Source: CAD feature listing. Evaluate the final solid. Frame: model axes, mm. Face numbers are marked on the shaded views. A direction names the side the tool comes from. Coordinates: 2 decimals unless noted, no trailing zeros. Order: outer loops, then holes, each group sorted by start corner. A loop starts at its lowest first (then second) coordinate and runs counter-clockwise, first axis right, second up. Notation, with made-up numbers: (49, 28.25) - (85, 28.25) arc R31 cw to (85, 54.25) - close; hole circle Ø8 at (32, 21.5). An arc over 180 degrees is marked (long way). One line per question, with ' | ' between items.
Autodesk Inventor part; units mm, degrees
ref_plane "YZ Plane" through (0, 0, 0) normal (1, 0, 0) x (0, 1, 0)
ref_plane "XZ Plane" through (0, 0, 0) normal (0, 1, 0) x (-1, 0, 0)
ref_plane "XY Plane" through (0, 0, 0) normal (0, 0, 1) x (1, 0, 0)
sketch "Sketch2" plane through (0, 0, 0) normal (0, 0, 1) x (1, 0, 0)
  line L0 (4.2, -19.2857) -> (4.2, 20.7143)
  line L1 (4.2, -19.2857) -> (15, -19.2857)
  line L2 (15, -19.2857) -> (15, -8.3281)
  line L3 (15, -8.3281) -> (20.3713, -0.6476)
  line L4 (20.3713, -0.6476) -> (20.3713, 40.7143)
  line L5 (20.3713, 40.7143) -> (0, 40.7143)
  line L6 (0, 40.7143) -> (0, 20.7143)
  line L7 (0, 20.7143) -> (4.2, 20.7143)
  point P0 (0, 0)
  dimension "d3" = 4.2
  dimension "d4" = 10.8
  dimension "d5" = 60
  dimension "d6" = 20
revolve "Revolution1" add sketch "Sketch2" angle 360 about axis through (0, 40.7143, 0) along (0, -1, 0)
fillet "Fillet1" radius 6 2 edges at (-20.3713, -0.6476, 0) (-15, -8.3281, 0)
fillet "Fillet2" radius 5 1 edges at (-20.3713, 40.7143, 0)
properties part number "Top Knob"
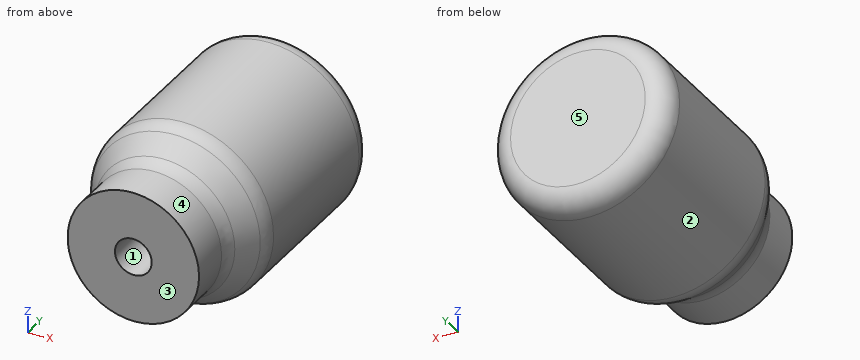
(1) Pull-direction query (Z, two-part tool) for the marked faces 1, 2 and 3; classes: pulls with the +Z half, pulls with the -Z half, needs draft (parallel to the pull), parting line crosses it, or undercut.
Taken from the geometry:
face 1: undercut | face 2: parting line crosses it | face 3: needs draft
(2) Material intervals for L1, parallel to Z at x = 0, y = -10; L2, parallel to Z at x = 0, y = 5; L3, parallel to X at y = -1, z = 2.5, sorted ascending. Write a range as from..to.
Taken from the geometry:
L1: z = -15..-4.2, 4.2..15 | L2: z = -20.37..-4.2, 4.2..20.37 | L3: x = -19.78..-3.37, 3.37..19.78
(3) Cut plane B-B (y = 33.5). Return the cut outline in (x, z).
Taken from the geometry:
outline: circle Ø40.74 at (0, 0)
(4) Set-up query: the marked faces 4 and 5. Return all of +Z, -Z, +X, -X, +Y, -Y with unobstructed straight access to the full face (end or side cutting, diameter ignored); none if empty.
Taken from the geometry:
face 4: -Y | face 5: +Z, -Z, +X, -X, +Y
(5) Pin query (flat end, axial travel): P1, Ø8, axis at x = -15, y = -5, coming from the -Z side; P2, Ø6.5, axis at x = 0, z = 0, coming from the -Y side; P3, Ø8, axis at y = -8, z = -3, coming from the -X side. Return the tip coordinate at first contact, or that it passes through.
Taken from the geometry:
P1: stops at z = -14.99 | P2: stops at y = 20.71 | P3: stops at x = -17.84
(6) Cut plane C-C (y = 8.5). Return the cut outline in (x, z).
Taken from the geometry:
outline: circle Ø40.74 at (0, 0); hole circle Ø8.4 at (0, 0)
(7) Cut plane A-A (y = -12). Return the cut outline in (x, z), and give its area (3 significant figures).
Taken from the geometry:
outline: circle Ø30 at (0, 0); hole circle Ø8.4 at (0, 0) | area: 651 mm²
